Can you work these out from the model? Positions are in its coordinate system, mm. A direction names the side the tool comes from. Coordinates: 2 decimals unless noted, no trailing zeros. Write each loop counter-clockwise with the first axis right and the second up, starting at its lowest first coordinate (ties: lowest second). Pieces come first, ordered by that corner, then holes. Notation, with made-up numbers: (77.5, 48) - (92.5, 48) arc R30 ccw to (92.5, 85) - close; hole circle Ø7 at (4.5, -17.75). An arc over 180 degrees is marked (long way). Write each question's results on one line, items separated by ' | '. Start each with the question number.
```python
from build123d import *

# Parameters (mm, degrees)
SKETCH_1_R          = 50
EXTRUDE_1_DEPTH     = 25
SKETCH_3_W          = 50
SKETCH_3_H          = 20
CUT_EXTRUDE_1_DEPTH = 20
SKETCH_6_W          = 25
SKETCH_6_H          = 5
EXTRUDE_2_DEPTH     = 15
EXTRUDE_3_DEPTH     = 5
SKETCH_7_R          = 2.5
CUT_EXTRUDE_2_DEPTH = 91.311959341
SKETCH_9_W          = 137.55999238
SKETCH_9_H          = 30
CUT_EXTRUDE_3_DEPTH = 20
CUT_EXTRUDE_4_DEPTH = 78.821912081


with BuildPart() as part:
    # 草圖1 → 填料-伸長1 (new body)
    with BuildSketch(Plane.XY):
        Circle(SKETCH_1_R)
    extrude(amount=EXTRUDE_1_DEPTH)

    # 草圖3 → 除料-伸長1 (cut)
    with BuildSketch(Plane(origin=(0, 0, 0), x_dir=(-1, 0, 0), z_dir=(0, 0, -1))):
        with Locations((0, 30)):
            Rectangle(SKETCH_3_W, SKETCH_3_H)
        with Locations((0, -30)):
            Rectangle(SKETCH_3_W, SKETCH_3_H)
    extrude(amount=-CUT_EXTRUDE_1_DEPTH, mode=Mode.SUBTRACT)

    # 草圖6 → 填料-伸長2 (add)
    with BuildSketch(Plane(origin=(0, 0, 0), x_dir=(-1, 0, 0), z_dir=(0, 0, -1))):
        with Locations((0, 17.5)):
            Rectangle(SKETCH_6_W, SKETCH_6_H)
        with Locations((0, -17.5)):
            Rectangle(SKETCH_6_W, SKETCH_6_H)
    extrude(amount=EXTRUDE_2_DEPTH)

    # 草圖8 → 填料-伸長3 (add)
    with BuildSketch(Plane.XZ.offset(20)):
        with BuildLine():
            Line((-12.5, -15), (12.5, -15))
            ThreePointArc((12.5, -15), (0, -27.5), (-12.5, -15))
        make_face()
    extrude_3 = extrude(amount=-EXTRUDE_3_DEPTH)

    # 鏡射1: 填料-伸長3 across plane
    add(extrude_3.mirror(Plane.ZX))

    # 草圖7 → 除料-伸長2 (cut, through all)
    with BuildSketch(Plane(origin=(0, 20, 0), x_dir=(1, 0, 0), z_dir=(0, 1, 0))):
        with Locations(Location((0, 12.5, 0), (0, 0, 270))):
            Circle(SKETCH_7_R)
    extrude(amount=-CUT_EXTRUDE_2_DEPTH, mode=Mode.SUBTRACT)

    # 草圖9 → 除料-伸長3 (cut)
    with BuildSketch(Plane.XY.offset(25)):
        with Locations((-0.331949789, 0)):
            Rectangle(SKETCH_9_W, SKETCH_9_H)
    extrude(amount=-CUT_EXTRUDE_3_DEPTH, mode=Mode.SUBTRACT)

    # 草圖10 → 除料-伸長4 (cut, through all)
    with BuildSketch(Plane.XY.offset(5)):
        with BuildLine():
            Line((-36.282162368, 9.958493657), (-36.282162368, -8.232354756))
            ThreePointArc((-36.282162368, -8.232354756), (-40, -11.950192388), (-43.717837632, -8.232354756))
            Line((-43.717837632, -8.232354756), (-43.717837632, 9.958493657))
            ThreePointArc((-43.717837632, 9.958493657), (-40, 13.676331289), (-36.282162368, 9.958493657))
        make_face()
        with BuildLine():
            Line((36.282162368, 9.958493657), (36.282162368, -8.232354756))
            ThreePointArc((36.282162368, -8.232354756), (40, -11.950192388), (43.717837632, -8.232354756))
            Line((43.717837632, -8.232354756), (43.717837632, 9.958493657))
            ThreePointArc((43.717837632, 9.958493657), (40, 13.676331289), (36.282162368, 9.958493657))
        make_face()
    extrude(amount=-CUT_EXTRUDE_4_DEPTH, mode=Mode.SUBTRACT)


solid = part.part
```
Q1. If we section it at A-A (y = 0): Please give me the cut outline in (x, z), then the cut area to 3 significant figures.
Q2. I need wall thicknesses on line 1 along X through (y, z) = (18.1, -12.5); line 2 along Y through (x, z) = (-4, -0.5); line 3 along X through (y, z) = (-9, 1.5). Which ranges of each line are inside material? Lowest first, please. Write a range as from..to.
Q3. I'm going to push flat-ended pins straight in: pin 1 Ø14 at (x, z) = (1.5, 3.5) entering from +Y; pin 2 Ø4 at (y, z) = (-37, 11.5) entering from +X; pin 3 Ø1.5 at (x, y) = (-36.5, 1) entering from +Z. Where does each tip first touch, or does it pass through?
Q4. For faces 4 (the face through (3, -15, -14)), 5 (the face through (40.082, 13.675, 2.535)), 6 (the face through (-12.5, -18, -7)), 7 (the face through (-1, 0, 5)), 8 (the face through (0, -20, 2)), which set-ups out of +Z, -Z, +X, -X, +Y, -Y let a thin tool reach every point of the face, with its end or its side?
Q5. Thinking about a two-plate mould opening in X: for faces 1 (the face through (-12.5, 17, -7)), 2 (the face through (12.5, -18, -7)), 3 (the face through (0, 40, 10)), which applies, pulls with the +X half, pulls with the -X half, needs draft (parallel to the pull), parting line crosses it, or undercut?
Q6. If we section it at D-D (x = -40): Please give me the cut outline in (y, z), then the cut area to 3 significant figures.
Q7. If we section it at C-C (x = 0): Please give me the cut outline in (y, z).
Q8. If we section it at B-B (z = -12.5): Please give me the cut outline in (x, y).
Answer list:
1) outline: (-50, 0) - (-43.72, 0) - (-43.72, 5) - (-50, 5) - close; (-36.28, 0) - (36.28, 0) - (36.28, 5) - (-36.28, 5) - close; (43.72, 0) - (50, 0) - (50, 5) - (43.72, 5) - close | area: 426 mm2
2) line 1: x = -12.5..-2.5, 2.5..12.5 | line 2: y = -20..-15, 15..20 | line 3: x = -49.18..-43.64, -36.36..36.36, 43.64..49.18
3) pin 1: stops at y = 50 | pin 2: stops at x = 35.71 | pin 3: stops at z = 5
4) face 4: -Z, +X, -X | face 5: +Z, -Z | face 6: -Z, -X, +Y, -Y | face 7: +Z, +X, -X | face 8: -Z
5) face 1: pulls with the -X half | face 2: pulls with the +X half | face 3: undercut
6) outline: (-30, 0) - (-11.95, 0) - (-11.95, 5) - (-15, 5) - (-15, 25) - (-30, 25) - close; (13.68, 0) - (30, 0) - (30, 25) - (15, 25) - (15, 5) - (13.68, 5) - close | area: 772 mm2
7) outline: (-50, 0) - (-40, 0) - (-40, 20) - (-20, 20) - (-20, -10) - (-15, -10) - (-15, 0) - (15, 0) - (15, -10) - (20, -10) - (20, 20) - (40, 20) - (40, 0) - (50, 0) - (50, 25) - (15, 25) - (15, 5) - (-15, 5) - (-15, 25) - (-50, 25) - close; (-20, -27.5) - (-15, -27.5) - (-15, -15) - (-20, -15) - close; (15, -27.5) - (20, -27.5) - (20, -15) - (15, -15) - close
8) outline: (-12.5, -20) - (-2.5, -20) - (-2.5, -15) - (-12.5, -15) - close; (-12.5, 15) - (-2.5, 15) - (-2.5, 20) - (-12.5, 20) - close; (2.5, -20) - (12.5, -20) - (12.5, -15) - (2.5, -15) - close; (2.5, 15) - (12.5, 15) - (12.5, 20) - (2.5, 20) - close
